Model file for the job. Use its own axes, mm. Give positions to 0.01 mm unless a question says otherwise; leave off trailing zeros. Loops run counter-clockwise (first coordinate to the right, second up) from the corner with the lowest first, then second, coordinate; pieces in that order, holes last. Notation, with made-up numbers: (29, 21) - (85, 21) arc R15 cw to (85, 32) - close; hole circle Ø7 at (5.5, -19.75). An arc over 180 degrees is marked (long way). Use a Markdown table: item, result.
Autodesk Inventor part; units mm, degrees
ref_plane "YZ Plane" through (0, 0, 0) normal (1, 0, 0) x (0, 1, 0)
ref_plane "XZ Plane" through (0, 0, 0) normal (0, 1, 0) x (-1, 0, 0)
ref_plane "XY Plane" through (0, 0, 0) normal (0, 0, 1) x (1, 0, 0)
sketch "Skizze1" plane through (0, 0, 0) normal (0, 0, 1) x (1, 0, 0)
  circle A0 centre (2.85, 15) radius 0.7835
  line L0 (0, 0) -> (5.7, 0)
  line L1 (5.7, 0) -> (5.7, 30)
  line L2 (0, 30) -> (5.7, 30)
  line L3 (0, 0) -> (0, 30)
extrude "Extrusion1" add sketch "Skizze1" along normal blind 2
chamfer "Fasen1" distance 1.7 angle 45 1 edges at (2.0665, 15, 2)
properties part number "LagerHH" material "Polyethylen, hohe Dichte, Gleitfläche"
(1) Drill centre lines: probe 1 along Y at (x, z) = (2.85, 0.2); probe 2 along Y at (x, z) = (3.85, 1.85); probe 3 along Z at (x, y) = (3.1, 13.75). Where is each one in solid material? Low to high. Write a range as [from, to].
Computed:
| item | result |
|---|---|
| probe 1 | [0, 14.22], [15.78, 30] |
| probe 2 | [0, 12.89], [17.11, 30] |
| probe 3 | [0, 0.79] |
(2) Mould opens along Y. For faces 1 (the flat face through (5.7, 15, 1)), 2 (the conical face through (3.7, 15.27, 0.41)), 3 (the flat face through (3, 0, 1)), 4 (the flat face through (3, 30, 1)) say: pulls with the +Y half, pulls with the -Y half, needs draft (parallel to the pull), parting line crosses it, or undercut.
Computed:
| item | result |
|---|---|
| face 1 | needs draft |
| face 2 | undercut |
| face 3 | pulls with the -Y half |
| face 4 | pulls with the +Y half |
(3) Slice it at C-C, the plane z = 1.55. Write the cut outline in (x, y).
Computed:
| item | result |
|---|---|
| outline | (0, 0) - (5.7, 0) - (5.7, 30) - (0, 30) - close; hole circle Ø4.07 at (2.85, 15) |
(4) Slice it at A-A, the plane y = 15. Write the cut outline in (x, z).
Computed:
| item | result |
|---|---|
| outline | (0, 0) - (2.07, 0) - (2.07, 0.3) - (0.37, 2) - (0, 2) - close; (3.63, 0) - (5.7, 0) - (5.7, 2) - (5.33, 2) - (3.63, 0.3) - close |
(5) Slice it at B-B, the plane x = 2.85. Write the cut outline in (y, z), plus the area to 3 significant figures.
Computed:
| item | result |
|---|---|
| outline | (0, 0) - (14.22, 0) - (14.22, 0.3) - (12.52, 2) - (0, 2) - close; (15.78, 0) - (30, 0) - (30, 2) - (17.48, 2) - (15.78, 0.3) - close |
| area | 54.0 mm² |
